from build123d import *

# Parameters (mm, degrees)
F1_DEPTH = 48.006
F2_DEPTH = 12.7


with BuildPart() as f1:
    # F0 (on Top) → F1 (new body)
    with BuildSketch(Plane.XY):
        with BuildLine():
            ThreePointArc((-29.534948, 0), (-38.834308, 22.45064), (-61.284948, 31.75))
            Line((-61.284948, 31.75), (-61.284948, 12.7))
            ThreePointArc((-61.284948, 12.7), (-52.304692, 8.980256), (-48.584948, 0))
            ThreePointArc((-48.584948, 0), (-52.304692, -8.980256), (-61.284948, -12.7))
            Line((-61.284948, -12.7), (-61.284948, -31.75))
            ThreePointArc((-61.284948, -31.75), (-38.834308, -22.45064), (-29.534948, 0))
        make_face()
        with BuildLine():
            Line((-61.284948, 12.7), (-61.284948, 31.75))
            ThreePointArc((-61.284948, 31.75), (-93.034948, 0), (-61.284948, -31.75))
            Line((-61.284948, -31.75), (-61.284948, -12.7))
            ThreePointArc((-61.284948, -12.7), (-73.984948, 0), (-61.284948, 12.7))
        make_face()
    extrude(amount=F1_DEPTH)

    # F0 (on Top) → F2 (join)
    with BuildSketch(Plane.XY):
        with BuildLine():
            Line((14.915052, 31.75), (-61.284948, 31.75))
            ThreePointArc((-61.284948, 31.75), (-38.834308, 22.45064), (-29.534948, 0))
            ThreePointArc((-29.534948, 0), (-38.834308, -22.45064), (-61.284948, -31.75))
            Line((-61.284948, -31.75), (14.915052, -31.75))
            Line((14.915052, -31.75), (14.915052, 31.75))
        make_face()
    extrude(amount=F2_DEPTH)


solid = f1.part
Here's how the part is built. I have some questions about the finished solid (model axes, mm). Coordinates: 2 decimals unless noted, no trailing zeros. Order: outer loops, then holes, each group sorted by start corner. A loop starts at its lowest first (then second) coordinate and runs counter-clockwise, first axis right, second up.
Item 1: If we section it at D-D on x = -3.5: List the corners of the cut face in (y, z) for me.
Result sheet:
outline: (-31.75, 0) - (31.75, 0) - (31.75, 12.7) - (-31.75, 12.7) - close
Item 2: If we section it at A-A on y = 9: List the corners of the cut face in (x, z) for me.
Result sheet:
outline: (-91.73, 0) - (-70.25, 0) - (-70.25, 48.01) - (-91.73, 48.01) - close; (-52.32, 0) - (14.92, 0) - (14.92, 12.7) - (-30.84, 12.7) - (-30.84, 48.01) - (-52.32, 48.01) - close
Item 3: If we section it at C-C on x = -62.5: List the corners of the cut face in (y, z) for me.
Result sheet:
outline: (-31.73, 0) - (-12.64, 0) - (-12.64, 48.01) - (-31.73, 48.01) - close; (12.64, 0) - (31.73, 0) - (31.73, 48.01) - (12.64, 48.01) - close
Item 4: I need wall thicknesses on line 1 (Z direction, x = -23.5, y = 27); line 2 (X direction, y = 10, z = 43.5); line 3 (Y direction, x = -57, z = 17.5). Which ranges of each line are inside material? Lowest first, please.
Result sheet:
line 1: z = 0 to 12.7
line 2: x = -91.42 to -69.11, -53.46 to -31.15
line 3: y = -31.46 to -11.96, 11.96 to 31.46
Item 5: If we section it at B-B on z = 6: List the corners of the cut face in (x, y) for me, plus the area to 3 significant figures.
Result sheet:
outline: (-61.28, -31.75) - (14.92, -31.75) - (14.92, 31.75) - (-61.28, 31.75) arc R31.75 ccw to start; hole circle Ø25.4 at (-61.28, 0)
area: 5,920 mm2
Item 6: For P1, Ø2, axis at x = -75.5, z = 37.5, coming from the -Y side; P2, Ø12, axis at x = -49, z = 20, coming from the +Y side; P3, Ø12, axis at y = -23.5, z = 25.5, coming from the +X side, each with a flat end and sliding along its axis, tell me the tip position at first contact or that it passes through.
Result sheet:
P1: stops at y = -28.87
P2: stops at y = 31.12
P3: stops at x = -34.79
